```python
from build123d import *

# Parameters (mm, degrees)
SKETCH2_R           = 97.45
SKETCH2_R_2         = 5.05
BOSS_EXTRUDE1_DEPTH = 5


with BuildPart() as part:
    # Sketch2 → Boss-Extrude1 (new body)
    with BuildSketch(Plane(origin=(0, 0, 0), x_dir=(1, 0, 0), z_dir=(0, 1, 0))):
        Circle(SKETCH2_R)
        with Locations((-34.05882548, -82.225278394)):
            Circle(SKETCH2_R_2, mode=Mode.SUBTRACT)
        with Locations((-82.225278394, -34.05882548)):
            Circle(SKETCH2_R_2, mode=Mode.SUBTRACT)
        with Locations((34.05882548, -82.225278394)):
            Circle(SKETCH2_R_2, mode=Mode.SUBTRACT)
        with Locations((82.225278394, -34.05882548)):
            Circle(SKETCH2_R_2, mode=Mode.SUBTRACT)
        with Locations((-82.225278394, 34.05882548)):
            Circle(SKETCH2_R_2, mode=Mode.SUBTRACT)
        with Locations((-34.05882548, 82.225278394)):
            Circle(SKETCH2_R_2, mode=Mode.SUBTRACT)
        with BuildLine():
            ThreePointArc((-64.431819773, -29.825167238), (-78.638188145, -16.488652353), (-70.985573699, 1.431197639))
            ThreePointArc((-70.985573699, 1.431197639), (-59.126750062, 39.306836901), (-28.79218644, 64.9))
            ThreePointArc((-28.79218644, 64.9), (0, 80), (28.79218644, 64.9))
            ThreePointArc((28.79218644, 64.9), (59.126750062, 39.306836901), (70.985573699, 1.431197639))
            ThreePointArc((70.985573699, 1.431197639), (78.638188145, -16.488652353), (64.431819773, -29.825167238))
            ThreePointArc((64.431819773, -29.825167238), (49.802006053, -50.603954323), (28.79218644, -64.9))
            ThreePointArc((28.79218644, -64.9), (0, -80), (-28.79218644, -64.9))
            ThreePointArc((-28.79218644, -64.9), (-49.802006053, -50.603954323), (-64.431819773, -29.825167238))
        make_face(mode=Mode.SUBTRACT)
        with Locations((82.225278394, 34.05882548)):
            Circle(SKETCH2_R_2, mode=Mode.SUBTRACT)
        with Locations((34.05882548, 82.225278394)):
            Circle(SKETCH2_R_2, mode=Mode.SUBTRACT)
    extrude(amount=BOSS_EXTRUDE1_DEPTH)


solid = part.part
```
Part model, mm, in its own coordinate system. A direction names the side the tool comes from. Round coordinates to 2 decimals unless told otherwise and drop trailing zeros. Write each loop counter-clockwise with the first axis right and the second up, starting at its lowest first coordinate (ties: lowest second). Pieces come first, ordered by that corner, then holes.
Item 1: Cut at D-D, the plane x = 35. Give the cut face in (y, z), plus the area to 3 significant figures.
Results:
outline: (0, -90.95) - (5, -90.95) - (5, -87.19) - (0, -87.19) - close; (0, -77.26) - (5, -77.26) - (5, -61.77) - (0, -61.77) - close; (0, 61.77) - (5, 61.77) - (5, 77.26) - (0, 77.26) - close; (0, 87.19) - (5, 87.19) - (5, 90.95) - (0, 90.95) - close
area: 193 mm2
Item 2: Two-plate mould, pull along Z, no slides. Class faces 1 (the cylindrical face through (-77.33, 2.46, 59.3)), 2 (the cylindrical face through (0, 2, 80)), 3 (the flat face through (-44, 0, -58)): +Z half, -Z half, draft (parallel to the pull), parting line (faces both ways), or undercut.
Results:
face 1: parting line
face 2: undercut
face 3: draft
Item 3: Cut at B-B, the plane z = 15. Give the cut face in (x, y).
Results:
outline: (-96.29, 0) - (-78.88, 0) - (-78.88, 5) - (-96.29, 5) - close; (78.88, 0) - (96.29, 0) - (96.29, 5) - (78.88, 5) - close
Item 4: Cut at C-C, the plane y = 1.5. Count the separate pieces of the cut face and the enclosed holes in it, plus the area to 3 significant figures.
Results:
separate pieces: 1
enclosed holes: 9
area: 12,200 mm2
Item 5: Which spindle directions (+Z, -Z, +X, -X, +Y, -Y) get a long thin tool onto all of the face, cutting with end or side? Do faces 4 (the flat face through (-44, 5, -58)), 5 (the cylindrical face through (78.695, 2.465, 16.204)). Say none if no direction does.
Results:
face 4: +Z, -Z, +X, -X, +Y
face 5: +Y, -Y
Item 6: Drop flat-ended pins along their axis: pin 1 Ø13 at (x, z) = (34.06, -82.23) entering from +Y; pin 2 Ø1.5 at (x, y) = (-24.5, 1) entering from -Z. Give the stop position or say it passes through.
Results:
pin 1: stops at y = 5
pin 2: stops at z = -94.51
Item 7: Probe L1, parallel to Z at x = -0.5, y = 1.9; L2, parallel to X at y = 3.4, z = 35; L3, parallel to X at y = 1.5, z = -31.5. List the from-to ranges inside material, lowest first.
Results:
L1: z = -97.45 to -80, 80 to 97.45
L2: x = -90.95 to -87.19, -77.26 to -61.77, 61.77 to 77.26, 87.19 to 90.95
L3: x = -92.22 to -86.58, -77.87 to -63.63, 63.63 to 77.87, 86.58 to 92.22
Item 8: Cut at A-A, the plane x = 0. Give the cut face in (y, z), plus the area to 4 significant figures.
Results:
outline: (0, -97.45) - (5, -97.45) - (5, -80) - (0, -80) - close; (0, 80) - (5, 80) - (5, 97.45) - (0, 97.45) - close
area: 174.5 mm2
